```python
from build123d import *

# Parameters (mm, degrees)
SKETCH1_W           = 18
SKETCH1_H           = 18
BOSS_EXTRUDE1_DEPTH = 2
SKETCH2_R           = 1.5
CUT_EXTRUDE1_DEPTH  = 2
SKETCH3_W           = 2
SKETCH3_H           = 10
BOSS_EXTRUDE2_DEPTH = 9


with BuildPart() as part:
    # Sketch1 → Boss-Extrude1 (new body)
    with BuildSketch(Plane(origin=(0, 0, 0), x_dir=(1, 0, 0), z_dir=(0, 1, 0))):
        with Locations((9, -9)):
            Rectangle(SKETCH1_W, SKETCH1_H)
    extrude(amount=BOSS_EXTRUDE1_DEPTH)

    # Sketch2 → Cut-Extrude1 (cut)
    with BuildSketch(Plane(origin=(0, 2, 0), x_dir=(1, 0, 0), z_dir=(0, 1, 0))):
        with Locations(Location((2.5, -2.5, 0), (0, 0, 270))):
            Circle(SKETCH2_R)
        with Locations(Location((15.5, -2.5, 0), (0, 0, 270))):
            Circle(SKETCH2_R)
    extrude(amount=-CUT_EXTRUDE1_DEPTH, mode=Mode.SUBTRACT)

    # Sketch3 → Boss-Extrude2 (add)
    with BuildSketch(Plane(origin=(0, 2, 0), x_dir=(1, 0, 0), z_dir=(0, 1, 0))):
        with Locations((1.5, -12)):
            Rectangle(SKETCH3_W, SKETCH3_H)
        with Locations((16.5, -12)):
            Rectangle(SKETCH3_W, SKETCH3_H)
    extrude(amount=BOSS_EXTRUDE2_DEPTH)


solid = part.part
```
Input: part model. Units: mm. Frame: model coordinates. A direction names the side the tool comes from. Coordinates: 2 decimals unless noted, no trailing zeros. Loops run counter-clockwise (first coordinate to the right, second up) from the corner with the lowest first, then second, coordinate; pieces in that order, holes last. Notation, with made-up numbers: M 11,-29 L 42,-29 A17 ccw 42,0 Z; hole C 46,-4.5 d9. An arc over 180 degrees is marked long. Answer in a Markdown table with one row per item.
1. Section D-D, the plane z = 13.75. Output: boundary loops of the cut face in (x, y).
Response:
| item | result |
|---|---|
| outline | M 0,0 L 18,0 L 18,2 L 17.5,2 L 17.5,11 L 15.5,11 L 15.5,2 L 2.5,2 L 2.5,11 L 0.5,11 L 0.5,2 L 0,2 Z |
2. First-contact query: pin 1 (0.6 mm diameter, centred on x = 1.5, y = 8.5, fed in from +Z); pin 2 (2.5 mm diameter, centred on y = 4.5, z = 14, fed in from +X); pin 3 (1.5 mm diameter, centred on y = 9, z = 12, fed in from -X). Flat tips, straight axial feed; report the tip coordinate or a pass-through.
Response:
| item | result |
|---|---|
| pin 1 | stops at z = 17 |
| pin 2 | stops at x = 17.5 |
| pin 3 | stops at x = 0.5 |
3. Section A-A, the plane y = 9.75. Output: boundary loops of the cut face in (x, z).
Response:
| item | result |
|---|---|
| outline | M 0.5,7 L 2.5,7 L 2.5,17 L 0.5,17 Z; M 15.5,7 L 17.5,7 L 17.5,17 L 15.5,17 Z |
4. Material intervals for line 1 (X direction, y = 1.2, z = 2.5); line 2 (X direction, y = 5.25, z = 9.5); line 3 (Y direction, x = 8.5, z = 9.75), sorted ascending.
Response:
| item | result |
|---|---|
| line 1 | x = 0 to 1, 4 to 14, 17 to 18 |
| line 2 | x = 0.5 to 2.5, 15.5 to 17.5 |
| line 3 | y = 0 to 2 |
5. Section B-B, the plane z = 2.5. Output: boundary loops of the cut face in (x, y), then the cut area to 3 significant figures.
Response:
| item | result |
|---|---|
| outline | M 0,0 L 1,0 L 1,2 L 0,2 Z; M 4,0 L 14,0 L 14,2 L 4,2 Z; M 17,0 L 18,0 L 18,2 L 17,2 Z |
| area | 24.0 mm2 |
6. Reachability of faces 1 (the flat face through (16, 6, 17)), 2 (the flat face through (0.5, 6, 12)), 3 (the flat face through (2.5, 6, 12)) from +Z, -Z, +X, -X, +Y, -Y: full face, straight path, thin tool, end or side. Return the list, or none.
Response:
| item | result |
|---|---|
| face 1 | +Z, +X, -X, +Y |
| face 2 | +Z, -Z, -X, +Y |
| face 3 | +Z, -Z, +Y |
7. Section C-C, the plane x = 16.25. Output: boundary loops of the cut face in (y, z).
Response:
| item | result |
|---|---|
| outline | M 0,0 L 2,0 L 2,1.2 L 0,1.2 Z; M 0,3.8 L 2,3.8 L 2,7 L 11,7 L 11,17 L 2,17 L 2,18 L 0,18 Z |
